Geometry: see drawing. Coordinates: mm, zero at the bounding-box minimum. Give positions to 0.01 mm unless a question says otherwise; leave off trailing zeros. Write each loop counter-clockwise with the first axis right and the second up, starting at its lowest first coordinate (ties: lowest second). Pieces come first, ordered by that corner, then holes. Notation, with made-up numbers: M 33,-2 L 43,-2 A8 ccw 43,12 Z; hole C 64,1.25 d10. An arc over 180 degrees is marked long. Use CSV: the item, a comma, the result in double quotes. Start each with the question number.
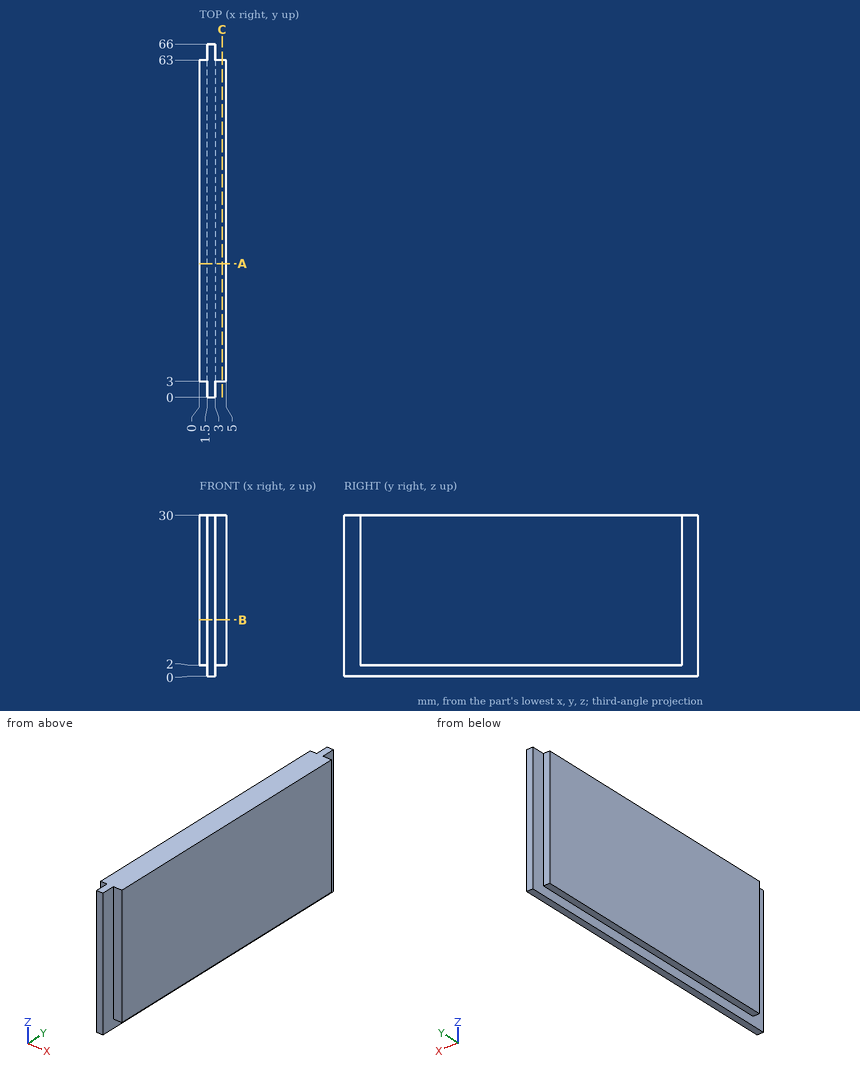
1. Section B-B on z = 10.5. Return loops of the section in (x, y).
2. Section C-C on x = 4.25. Return loops of the section in (y, z).
3. Line query: probe 1 along Y at (x, z) = (3.9, 2.5); probe 2 along Z at (x, y) = (4.1, 60.5). Output: solid intervals per line, ascending.
4. First-contact query: pin 1 (1.2 mm diameter, centred on x = 0.5, z = 22, fed in from +Y); pin 2 (1.2 mm diameter, centred on x = 0.5, z = 12.5, fed in from -Y). Flat tips, straight axial feed; report the tip coordinate or a pass-through.
5. Section A-A on y = 25. Return loops of the section in (x, z), then the cut area to 3 significant figures.
Resolved:
1,outline,"M 0,3 L 1.5,3 L 1.5,0 L 3,0 L 3,3 L 5,3 L 5,63 L 3,63 L 3,66 L 1.5,66 L 1.5,63 L 0,63 Z"
2,outline,"M 3,2 L 63,2 L 63,30 L 3,30 Z"
3,probe 1,"y = 3 to 63"
3,probe 2,"z = 2 to 30"
4,pin 1,"stops at y = 63"
4,pin 2,"stops at y = 3"
5,outline,"M 0,2 L 1.5,2 L 1.5,0 L 3,0 L 3,2 L 5,2 L 5,30 L 0,30 Z"
5,area,"143 mm2"
